Read the model definition and answer for the solid it produces. Units are mm, in the model's axes. A direction names the side the tool comes from. Round coordinates to 2 decimals unless told otherwise and drop trailing zeros. Write each loop counter-clockwise with the first axis right and the second up, starting at its lowest first coordinate (ties: lowest second). Pieces come first, ordered by that corner, then holes. Notation, with made-up numbers: (40, 30) -> (90, 30) arc R22 cw to (90, 51) -> close; hole circle Ø1 at (-35.75, 52). An arc over 180 degrees is marked (long way). Return JSON: item names as keys, results as strings. Group by question number.
(1) A cutting plane is placed at A-A on x = 0. Give the vertices of the cut face in (y, z), then the cut area to 4 significant figures.
(2) The mould has two halves that part along Z. Classify faces 1 (the flat face through (0, 3.75, 0)), 2 (the flat face through (0, -3, 0)), 3 (the flat face through (2.4, -0.1, -3.75)): released by +Z, released by -Z, zero draft, split by the parting line, or undercut.
(3) Given pin 1 (2.5 mm diameter, centred on x = 0, y = 0, fed in from +Z); pin 2 (3 mm diameter, centred on y = 1, z = -2, fed in from -X), each flat-ended and moving along its own axis, determine where each tip first touches the part or whether it passes through.
(4) A cutting plane is placed at D-D on y = 0. Give the vertices of the cut face in (x, z), then the cut area to 3 significant figures.
(5) A cutting plane is placed at B-B on y = 2.5. Give the vertices of the cut face in (x, z).
(6) For faces 4 (the flat face through (-10, -3.4, 0.1)), 5 (the flat face through (2.4, 0, 3)), determine the directions among +Z, -Z, +X, -X, +Y, -Y from which every point of the face is accessible in a straight line to the end or side of a thin tool.
(7) Straight lines are drawn through the part: line 1 (Z direction, x = 6.25, y = -0.25); line 2 (Y direction, x = 0, z = 3.2). For each, find the intervals that lie inside material, in ascending order.
```python
from build123d import *

# Parameters (mm, degrees)
F0_W     = 7.5
F0_H     = 7.5
F0_W_2   = 6
F0_H_2   = 6
F1_DEPTH = 10
F2_R     = 2
F3_DEPTH = 25


with BuildPart() as f1:
    # F0 (on Right) → F1 (new body, symmetric)
    with BuildSketch(Plane.YZ):
        Rectangle(F0_W, F0_H)
        Rectangle(F0_W_2, F0_H_2, mode=Mode.SUBTRACT)
    extrude(amount=F1_DEPTH, both=True)

    # F2 (on face) → F3 (cut)
    with BuildSketch(Plane.XY.offset(3.75)):
        Circle(F2_R)
    extrude(amount=-F3_DEPTH, mode=Mode.SUBTRACT)


solid = f1.part
```
Checks:
{
 "1": {"outline": "(-3.75, -3.75) -> (-2, -3.75) -> (-2, -3) -> (-3, -3) -> (-3, 3) -> (-2, 3) -> (-2, 3.75) -> (-3.75, 3.75) -> close; (2, -3.75) -> (3.75, -3.75) -> (3.75, 3.75) -> (2, 3.75) -> (2, 3) -> (3, 3) -> (3, -3) -> (2, -3) -> close", "area": "14.25 mm^2"},
 "2": {"face 1": "zero draft", "face 2": "undercut", "face 3": "released by -Z"},
 "3": {"pin 1": "passes through", "pin 2": "stops at x = -10"},
 "4": {"outline": "(-10, -3.75) -> (-2, -3.75) -> (-2, -3) -> (-10, -3) -> close; (-10, 3) -> (-2, 3) -> (-2, 3.75) -> (-10, 3.75) -> close; (2, -3.75) -> (10, -3.75) -> (10, -3) -> (2, -3) -> close; (2, 3) -> (10, 3) -> (10, 3.75) -> (2, 3.75) -> close", "area": "24.0 mm^2"},
 "5": {"outline": "(-10, -3.75) -> (10, -3.75) -> (10, -3) -> (-10, -3) -> close; (-10, 3) -> (10, 3) -> (10, 3.75) -> (-10, 3.75) -> close"},
 "6": {"face 4": "+Z, -Z, -X, +Y, -Y", "face 5": "+X, -X"},
 "7": {"line 1": "z = -3.75 to -3, 3 to 3.75", "line 2": "y = -3.75 to -2, 2 to 3.75"}
}
